```python
from build123d import *

# Parameters (mm, degrees)
SKETCH1_W                                = 53
SKETCH1_H                                = 26
BOSS_EXTRUDE1_DEPTH                      = 8
SKETCH2_W                                = 15.5
SKETCH2_H                                = 16
CUT_EXTRUDE1_DEPTH                       = 9
SKETCH3_W                                = 15.5
SKETCH3_H                                = 16
CUT_EXTRUDE2_DEPTH                       = 9
SKETCH4_W                                = 40.000000023
SKETCH4_H                                = 5
CUT_EXTRUDE3_DEPTH                       = 9
CBORE_FOR_M10_HEX_HEAD_BOLT1_D           = 11.4
CBORE_FOR_M10_HEX_HEAD_BOLT1_CBORE_D     = 16.2
CBORE_FOR_M10_HEX_HEAD_BOLT1_CBORE_DEPTH = 2
F_3_3_3_3_DIAMETER_HOLE1_D               = 3.3
F_3_3_3_3_DIAMETER_HOLE1_DEPTH           = 6
F_3_3_3_3_DIAMETER_HOLE1_TIP             = 0.991420021
FILLET1_R                                = 4
FILLET2_R                                = 5
CHAMFER1_SIZE                            = 8
CHAMFER1_SIZE2                           = 4
CHAMFER2_SIZE                            = 4
CHAMFER2_SIZE2                           = 8


with BuildPart() as part:
    # Sketch1 → Boss-Extrude1 (new body)
    with BuildSketch(Plane.XZ):
        with Locations((0, 13)):
            Rectangle(SKETCH1_W, SKETCH1_H)
    extrude(amount=-BOSS_EXTRUDE1_DEPTH)

    # Sketch2 → Cut-Extrude1 (cut, through all)
    with BuildSketch(Plane(origin=(0, 8, 0), x_dir=(-1, 0, 0), z_dir=(0, 1, 0))):
        with Locations((-18.75, 18)):
            Rectangle(SKETCH2_W, SKETCH2_H)
    extrude(amount=-CUT_EXTRUDE1_DEPTH, mode=Mode.SUBTRACT)

    # Sketch3 → Cut-Extrude2 (cut, through all)
    with BuildSketch(Plane(origin=(0, 8, 0), x_dir=(-1, 0, 0), z_dir=(0, 1, 0))):
        with Locations((18.75, 18)):
            Rectangle(SKETCH3_W, SKETCH3_H)
    extrude(amount=-CUT_EXTRUDE2_DEPTH, mode=Mode.SUBTRACT)

    # Sketch4 → Cut-Extrude3 (cut, through all)
    with BuildSketch(Plane(origin=(0, 8, 0), x_dir=(-1, 0, 0), z_dir=(0, 1, 0))):
        with Locations((1.2e-08, 2.5)):
            Rectangle(SKETCH4_W, SKETCH4_H)
    extrude(amount=-CUT_EXTRUDE3_DEPTH, mode=Mode.SUBTRACT)

    # CBORE for M10 Hex Head Bolt1 (through all)
    with Locations(Plane(origin=(0, 0, 0), x_dir=(-1, 0, 0), z_dir=(0, -1, 0))):
        with Locations((0, -15)):
            CounterBoreHole(CBORE_FOR_M10_HEX_HEAD_BOLT1_D / 2, CBORE_FOR_M10_HEX_HEAD_BOLT1_CBORE_D / 2, CBORE_FOR_M10_HEX_HEAD_BOLT1_CBORE_DEPTH)

    # Ø3.3 (3.3) Diameter Hole1
    with Locations(Plane(origin=(0, 0, 0), x_dir=(-1, 0, 0), z_dir=(0, 0, -1))):
        with Locations((-23.25, 4), (23.25, 4)):
            Hole(F_3_3_3_3_DIAMETER_HOLE1_D / 2, depth=F_3_3_3_3_DIAMETER_HOLE1_DEPTH)
            with Locations((0, 0, -(F_3_3_3_3_DIAMETER_HOLE1_DEPTH + F_3_3_3_3_DIAMETER_HOLE1_TIP / 2))):  # 118° drill point
                Cone(0, F_3_3_3_3_DIAMETER_HOLE1_D / 2, F_3_3_3_3_DIAMETER_HOLE1_TIP, mode=Mode.SUBTRACT)

    # Fillet1
    fillet1_edges = [part.edges().sort_by_distance(p)[0] for p in [
        (20, 4, 5),
        (-20.000000023, 4, 5),
    ]]
    fillet(fillet1_edges, radius=FILLET1_R)

    # Fillet2
    fillet2_edges = [part.edges().sort_by_distance(p)[0] for p in [
        (11, 4, 10),
        (11, 4, 26),
        (-11, 4, 26),
        (-11, 4, 10),
    ]]
    fillet(fillet2_edges, radius=FILLET2_R)

    # Chamfer1
    chamfer1_edges = [part.edges().sort_by_distance(p)[0] for p in [
        (-26.5, 4, 10),
    ]]
    chamfer1_side = [part.faces().sort_by_distance(p)[0] for p in [
        (-21.25, 4, 10),
    ]]
    chamfer(chamfer1_edges, length=CHAMFER1_SIZE, length2=CHAMFER1_SIZE2, reference=chamfer1_side[0])

    # Chamfer2
    chamfer2_edges = [part.edges().sort_by_distance(p)[0] for p in [
        (26.5, 4, 10),
    ]]
    chamfer2_side = [part.faces().sort_by_distance(p)[0] for p in [
        (26.5, 4, 5),
    ]]
    chamfer(chamfer2_edges, length=CHAMFER2_SIZE, length2=CHAMFER2_SIZE2, reference=chamfer2_side[0])


solid = part.part
```
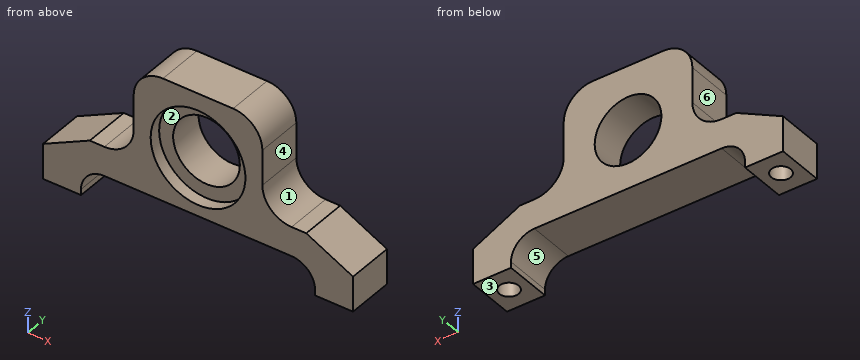
The model under review builds one solid part; all positions refer to its coordinate system, in mm. Face numbers are marked on the shaded views. A direction names the side the tool comes from. Round coordinates to 2 decimals unless told otherwise and drop trailing zeros. Loops run counter-clockwise (first coordinate to the right, second up) from the corner with the lowest first, then second, coordinate; pieces in that order, holes last. Notation, with made-up numbers: M 25.5,15 L 34.5,15 A21 cw 34.5,27 Z; hole C 2.25,-17 d11. An arc over 180 degrees is marked long. Answer as a JSON object with one key per item and string values.
(1) Clearance check with flat-ended pins moving along their axes: P1, Ø2, axis at x = -23.25, y = 4, coming from the -Z side; P2, Ø1, axis at x = 16, y = 3.5, coming from the -Z side; P3, Ø2, axis at x = 13, z = 13, coming from the +Y side; P4, Ø0.8, axis at x = -16.5, y = 3, coming from the +Z side. State where each tip first meets the part, or that it passes through.
Resolved:
{"P1": "z = 6.39", "P2": "z = 4.97", "P3": "through", "P4": "z = 10"}
(2) Tool access review of the marked faces 4, 5 and 6: name each direction out of +Z, -Z, +X, -X, +Y, -Y from which nothing blocks a thin tool from reaching the whole face with its end or side.
Resolved:
{"face 4": "+Z, +X, +Y, -Y", "face 5": "-Z, +Y, -Y", "face 6": "+Z, -X, +Y, -Y"}
(3) To check wall thickness, follow line 1 along Y through (x, z) = (23.25, 2.1); line 2 along X through (y, z) = (4, 2.3); line 3 along X through (y, z) = (4, 1.9). State the ranges of each line that lie inside material, in increasing order.
Resolved:
{"line 1": "0 to 2.35, 5.65 to 8", "line 2": "-26.5 to -24.9, -21.6 to -19.78, 19.78 to 21.6, 24.9 to 26.5", "line 3": "-26.5 to -24.9, -21.6 to -19.9, 19.9 to 21.6, 24.9 to 26.5"}
(4) Take a section at D-D on y = 7. Give the boundary of the cut face in (x, z), and give its area (3 significant figures).
Resolved:
{"outline": "M -26.5,0 L -20,0 L -20,1 A4 cw -16,5 L 16,5 A4 cw 20,1 L 20,0 L 26.5,0 L 26.5,6 L 18.5,10 L 16,10 A5 cw 11,15 L 11,21 A5 ccw 6,26 L -6,26 A5 ccw -11,21 L -11,15 A5 cw -16,10 L -18.5,10 L -26.5,6 Z; hole C 0,15 d11.4", "area": "555 mm²"}
(5) Take a section at A-A on x = 0. Give the boundary of the cut face in (y, z), and give its area (3 significant figures).
Resolved:
{"outline": "M 0,5 L 8,5 L 8,9.3 L 2,9.3 L 2,6.9 L 0,6.9 Z; M 0,23.1 L 2,23.1 L 2,20.7 L 8,20.7 L 8,26 L 0,26 Z", "area": "67.2 mm²"}
(6) Draft analysis for pull direction X (two halves, no side actions). For the marked faces 1, 2 and 3, state which applies: released by +X, released by -X, zero draft, split by the parting line, or undercut.
Resolved:
{"face 1": "released by +X", "face 2": "undercut", "face 3": "zero draft"}
(7) Take a section at C-C on z = 20. Give the boundary of the cut face in (x, y), and give its area (3 significant figures).
Resolved:
{"outline": "M -11,0 L -6.37,0 L -6.37,2 L -2.74,2 L -2.74,8 L -11,8 Z; M 2.74,2 L 6.37,2 L 6.37,0 L 11,0 L 11,8 L 2.74,8 Z", "area": "118 mm²"}
(8) Take a section at B-B on y = 1. Give the boundary of the cut face in (x, z), and give its area (3 significant figures).
Resolved:
{"outline": "M -26.5,0 L -20,0 L -20,1 A4 cw -16,5 L 16,5 A4 cw 20,1 L 20,0 L 26.5,0 L 26.5,6 L 18.5,10 L 16,10 A5 cw 11,15 L 11,21 A5 ccw 6,26 L -6,26 A5 ccw -11,21 L -11,15 A5 cw -16,10 L -18.5,10 L -26.5,6 Z; hole C 0,15 d16.2", "area": "451 mm²"}
